Could you check a few things on this model? Use its own coordinates, in mm. Face numbers are marked on the shaded views. A direction names the side the tool comes from. Round coordinates to 2 decimals unless told otherwise and drop trailing zeros. Loops run counter-clockwise (first coordinate to the right, second up) from the corner with the lowest first, then second, coordinate; pieces in that order, holes last. Notation, with made-up numbers: M -32,60 L 1,60 A23 cw 1,96 Z; hole C 12,3 d11. An arc over 180 degrees is marked long. Return JSON: item names as keys, results as strings. Group by question number.
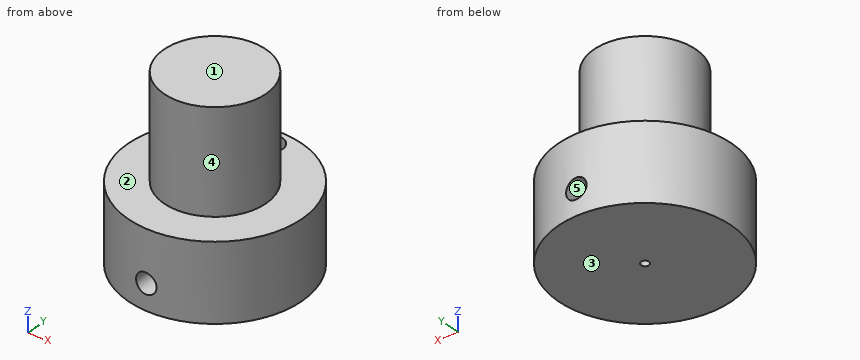
```python
from build123d import *

# Parameters (mm, degrees)
F0_R      = 17
F1_DEPTH  = 15
F2_R      = 10
F3_DEPTH  = 20
F4_R      = 0.8
F5_DEPTH  = 5
F7_R      = 2
F8_DEPTH  = 42.001
F9_R      = 2.5
F10_DEPTH = 5


with BuildPart() as f1:
    # F0 (on Top) → F1 (new body)
    with BuildSketch(Plane.XY):
        Circle(F0_R)
    extrude(amount=F1_DEPTH)

    # F2 (on face) → F3 (join)
    with BuildSketch(Plane.XY.offset(15)):
        Circle(F2_R)
    extrude(amount=F3_DEPTH)

    # F4 (on face) → F5 (cut)
    with BuildSketch(Plane(origin=(0, 0, 0), x_dir=(1, 0, 0), z_dir=(0, 0, -1))):
        Circle(F4_R)
    extrude(amount=-F5_DEPTH, mode=Mode.SUBTRACT)

    # F7 (on offset) → F8 (cut, through all)
    with BuildSketch(Plane.XZ.offset(25)):
        with Locations((0, 5)):
            Circle(F7_R)
    extrude(amount=-F8_DEPTH, mode=Mode.SUBTRACT)

    # F9 (on face) → F10 (cut)
    with BuildSketch(Plane.XY.offset(15)):
        with Locations((0, 13.5)):
            Circle(F9_R)
    extrude(amount=-F10_DEPTH, mode=Mode.SUBTRACT)


solid = f1.part
```
1. On a 3-axis mill with a long thin cutter (end or side, diameter ignored), from which of +Z, -Z, +X, -X, +Y, -Y can I reach the whole of each face in a straight line? I mean the marked faces 1 and 2. Say none if no direction works.
2. I'm going to push flat-ended pins straight in: pin 1 Ø1 at (x, z) = (11.5, 8.5) entering from +Y; pin 2 Ø10 at (x, y) = (6, -8) entering from -Z; pin 3 Ø1.5 at (x, y) = (-1, 13.5) entering from +Z; pin 4 Ø6 at (x, y) = (13, -10.5) entering from +Z. Where does each tip first touch, or does it pass through?
3. If we section it at C-C, the plane z = 5: Please give me the cut outline in (x, y).
4. If we section it at A-A, the plane x = 0: Please give me the cut outline in (y, z).
5. If we section it at B-B, the plane y = 7.5: Please give me the cut outline in (x, z), then the cut area to 3 significant figures.
6. I need wall thicknesses on probe 1 along Y at (x, z) = (0, 1.9); probe 2 along Z at (x, y) = (0, -8); probe 3 along Z at (x, y) = (-12.5, -6). Which ranges of each line are inside material? Lowest first, please.
7. We'd pull the mould along Z, two halves only. Please class the marked faces 3, 4 and 5: +Z half, -Z half, draft (parallel to the pull), parting line (faces both ways), or undercut.
8. If we section it at D-D, the plane y = 0: Please give me the cut outline in (x, z).
Geometry results:
{
 "1": {"face 1": "+Z, +X, -X, +Y, -Y", "face 2": "+Z"},
 "2": {"pin 1": "y = 12.96", "pin 2": "z = 0", "pin 3": "z = 10", "pin 4": "z = 15"},
 "3": {"outline": "M -2,-16.88 L -2,16.88 A17 ccw Z; M 2,-16.88 A17 ccw 2,16.88 Z"},
 "4": {"outline": "M -17,0 L -0.8,0 L -0.8,3 L -17,3 Z; M -17,7 L 17,7 L 17,15 L 16,15 L 16,10 L 11,10 L 11,15 L 10,15 L 10,35 L -10,35 L -10,15 L -17,15 Z; M 0.8,0 L 17,0 L 17,3 L 0.8,3 Z"},
 "5": {"outline": "M -15.26,0 L 15.26,0 L 15.26,15 L 6.61,15 L 6.61,35 L -6.61,35 L -6.61,15 L -15.26,15 Z; hole C 0,5 d4", "area": "710 mm^2"},
 "6": {"probe 1": "-17 to -0.8, 0.8 to 17", "probe 2": "0 to 3, 7 to 35", "probe 3": "0 to 15"},
 "7": {"face 3": "-Z half", "face 4": "draft", "face 5": "undercut"},
 "8": {"outline": "M -17,0 L -0.8,0 L -0.8,3.17 A2 cw long 0.8,3.17 L 0.8,0 L 17,0 L 17,15 L 10,15 L 10,35 L -10,35 L -10,15 L -17,15 Z"}
}
